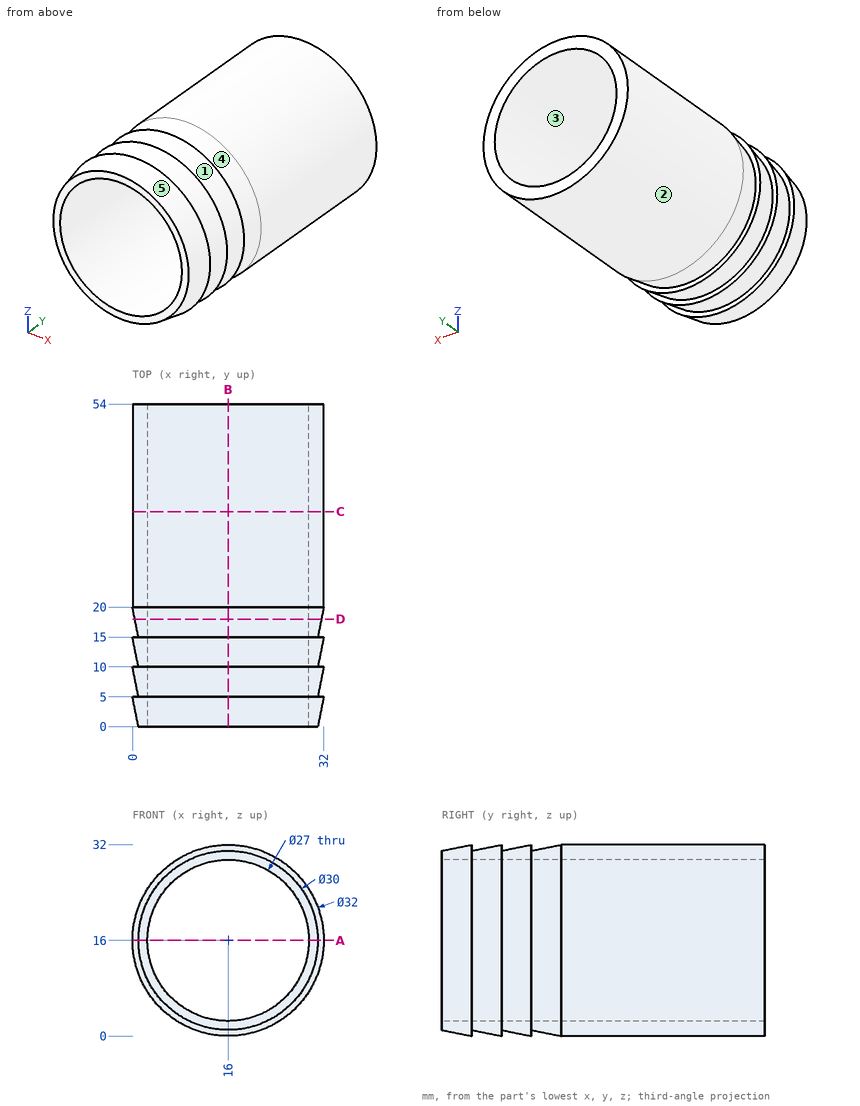
Here's the drawing with two shaded views (mm, measured from the low corner). I have some questions. A direction names the side the tool comes from. Round coordinates to 2 decimals unless told otherwise and drop trailing zeros. Loops run counter-clockwise (first coordinate to the right, second up) from the corner with the lowest first, then second, coordinate; pieces in that order, holes last. Notation, with made-up numbers: (-15.5, -5) - (-6.5, -5) arc R18 ccw to (-6.5, 4) - close; hole circle Ø6 at (28, 1.25). An arc over 180 degrees is marked (long way). Write item = value, one per line.
1) On a 3-axis mill with a long thin cutter (end or side, diameter ignored), from which of +Z, -Z, +X, -X, +Y, -Y can I reach the whole of each face in a straight line? I mean the marked faces 1 and 2. Say none if no direction works.
Computed:
face_1 = none
face_2 = +Y, -Y
2) Imagine slicing it at D-D (y = 18). Please give me the cut outline in (x, z), and give its area (3 significant figures).
Computed:
outline = circle Ø31.2 at (16, 16); hole circle Ø27 at (16, 16)
area = 192 mm2
3) If we mould it in two halves opening along Y, with no side actions, what happens to the marked faces 3, 4 and 5? For each: pulls with the +Y half, pulls with the -Y half, needs draft (parallel to the pull), parting line crosses it, or undercut.
Computed:
face_3 = needs draft
face_4 = undercut
face_5 = pulls with the -Y half
4) Imagine slicing it at C-C (y = 36). Please give me the cut outline in (x, z).
Computed:
outline = circle Ø32 at (16, 16); hole circle Ø27 at (16, 16)
5) Imagine slicing it at B-B (x = 16). Please give me the cut outline in (y, z), and give its area (3 significant figures).
Computed:
outline = (0, 1) - (5, 0) - (5, 1) - (10, 0) - (10, 1) - (15, 0) - (15, 1) - (20, 0) - (54, 0) - (54, 2.5) - (0, 2.5) - close; (0, 29.5) - (54, 29.5) - (54, 32) - (20, 32) - (15, 31) - (15, 32) - (10, 31) - (10, 32) - (5, 31) - (5, 32) - (0, 31) - close
area = 250 mm2
6) Imagine slicing it at A-A (z = 16). Please give me the cut outline in (x, y).
Computed:
outline = (0, 5) - (1, 0) - (2.5, 0) - (2.5, 54) - (0, 54) - (0, 20) - (1, 15) - (0, 15) - (1, 10) - (0, 10) - (1, 5) - close; (29.5, 0) - (31, 0) - (32, 5) - (31, 5) - (32, 10) - (31, 10) - (32, 15) - (31, 15) - (32, 20) - (32, 54) - (29.5, 54) - close
7) I'm going to push flat-ended pins straight in: P1, Ø5, axis at x = 27.5, y = 20.5, coming from the -Z side; P2, Ø12, axis at x = 27, z = 19, coming from the +Y side; P3, Ø4, axis at x = 6.5, y = 25, coming from the -Z side; P4, Ø6, axis at y = 10.5, z = 13, coming from the +X side. Where does each tip first touch, or does it pass through?
Computed:
P1 = 2.77
P2 = 54
P3 = 1.87
P4 = 32
8) I need wall thicknesses on line 1 along Z through (x, y) = (16, 33); line 2 along Z through (x, y) = (18.5, 11); line 3 along X through (y, z) = (39, 23). Which ranges of each line are inside material? Lowest first, please. Write a range as from..to.
Computed:
line_1 = 0..2.5, 29.5..32
line_2 = 1.01..2.73, 29.27..30.99
line_3 = 1.61..4.46, 27.54..30.39
